Source: three-view drawing plus pictorial views. Frame: mm from the lowest corner of the part. Round coordinates to 2 decimals unless told otherwise and drop trailing zeros. Write each loop counter-clockwise with the first axis right and the second up, starting at its lowest first coordinate (ties: lowest second). Pieces come first, ordered by that corner, then holes.
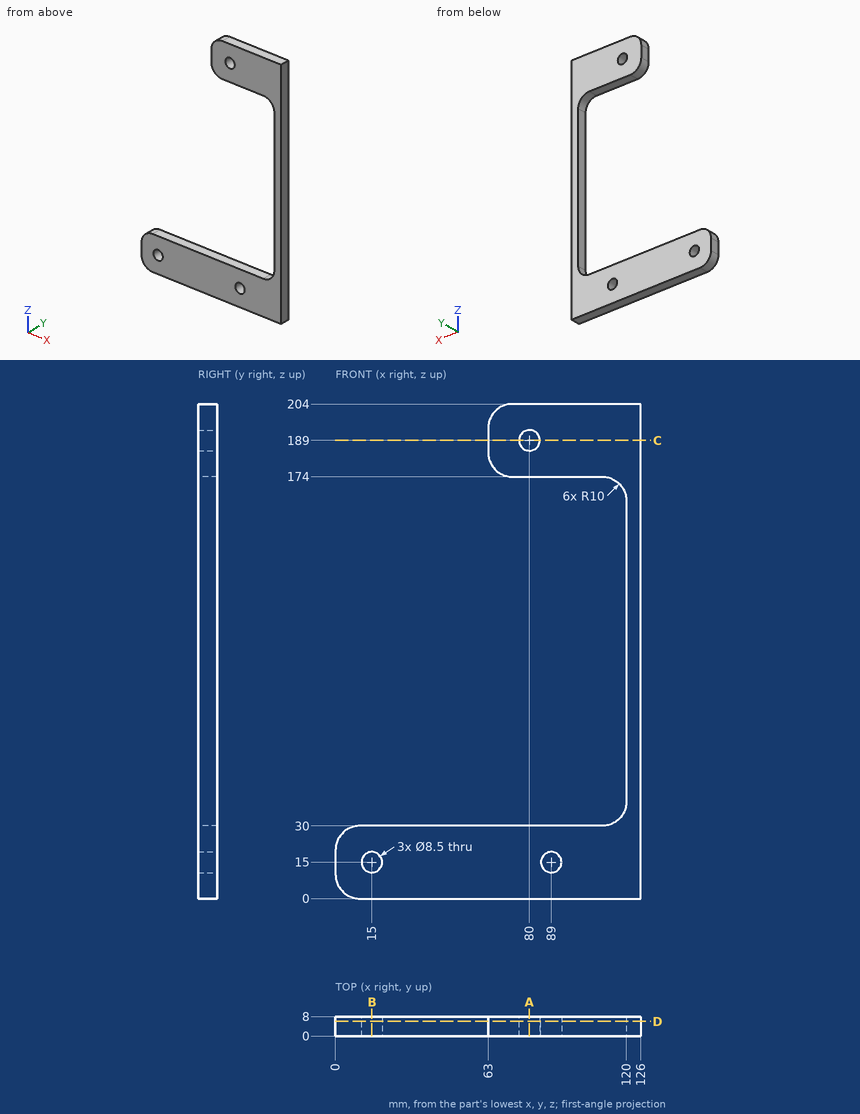
1) Line query: probe 1 along Z at (x, y) = (80, 5.5); probe 2 along Z at (x, y) = (89, 4.5); probe 3 along Z at (x, y) = (103.5, 4). Output: solid intervals per line, ascending.
2) Section D-D on y = 6. Output: boundary loops of the cut face in (x, z).
3) Section A-A on x = 80. Output: boundary loops of the cut face in (y, z), plus the area to 3 significant figures.
4) Section B-B on x = 15. Output: boundary loops of the cut face in (y, z).
5) First-contact query: P1, Ø4, axis at y = 4.5, z = 56, coming from the -X side; P2, Ø5, axis at x = 80, z = 189, coming from the -Y side; P3, Ø4, axis at y = 4, z = 190, coming from the -X side. Flat tips, straight axial feed; report the tip coordinate or a pass-through.
6) Section C-C on z = 189. Output: boundary loops of the cut face in (x, y), plus the area to 3 significant figures.
Filled in:
1. probe 1: z = 0 to 30, 174 to 184.75, 193.25 to 204
1. probe 2: z = 0 to 10.75, 19.25 to 30, 174 to 204
1. probe 3: z = 0 to 30, 174 to 204
2. outline: (0, 10) arc R10 ccw to (10, 0) - (126, 0) - (126, 204) - (73, 204) arc R10 ccw to (63, 194) - (63, 184) arc R10 ccw to (73, 174) - (110, 174) arc R10 cw to (120, 164) - (120, 40) arc R10 cw to (110, 30) - (10, 30) arc R10 ccw to (0, 20) - close; hole circle Ø8.5 at (15, 15); hole circle Ø8.5 at (80, 189); hole circle Ø8.5 at (89, 15)
3. outline: (0, 0) - (8, 0) - (8, 30) - (0, 30) - close; (0, 174) - (8, 174) - (8, 184.75) - (0, 184.75) - close; (0, 193.25) - (8, 193.25) - (8, 204) - (0, 204) - close
3. area: 412 mm2
4. outline: (0, 0) - (8, 0) - (8, 10.75) - (0, 10.75) - close; (0, 19.25) - (8, 19.25) - (8, 30) - (0, 30) - close
5. P1: stops at x = 120
5. P2: passes through
5. P3: stops at x = 63
6. outline: (63, 0) - (75.75, 0) - (75.75, 8) - (63, 8) - close; (84.25, 0) - (126, 0) - (126, 8) - (84.25, 8) - close
6. area: 436 mm2
